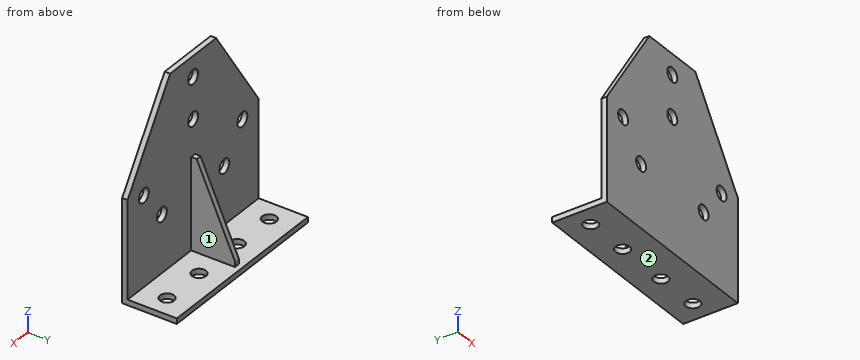
from build123d import *

# Parameters (mm, degrees)
SKETCH1_W      = 410
SKETCH1_H      = 120
SKETCH1_R      = 15.5
EXTRUDE1_DEPTH = 12
SKETCH2_W      = 410
SKETCH2_H      = 12
EXTRUDE2_DEPTH = 413
SKETCH3_R      = 15.5
EXTRUDE3_DEPTH = 413
SKETCH4_W      = 12
SKETCH4_H      = 96
EXTRUDE4_DEPTH = 200
EXTRUDE5_DEPTH = 200


with BuildPart() as part:
    # Sketch1 → Extrude1 (new body)
    with BuildSketch(Plane.XY):
        with Locations((205, 60)):
            Rectangle(SKETCH1_W, SKETCH1_H)
        with Locations((45, 67)):
            Circle(SKETCH1_R, mode=Mode.SUBTRACT)
        with Locations((145, 67)):
            Circle(SKETCH1_R, mode=Mode.SUBTRACT)
        with Locations((265, 67)):
            Circle(SKETCH1_R, mode=Mode.SUBTRACT)
        with Locations((365, 67)):
            Circle(SKETCH1_R, mode=Mode.SUBTRACT)
    extrude(amount=EXTRUDE1_DEPTH)

    # Sketch2 → Extrude2 (add)
    with BuildSketch(Plane.XY.offset(12)):
        with Locations((205, 6)):
            Rectangle(SKETCH2_W, SKETCH2_H)
    extrude(amount=EXTRUDE2_DEPTH)

    # Sketch3 → Extrude3 (cut)
    with BuildSketch(Plane(origin=(0, 12, 0), x_dir=(1, 0, 0), z_dir=(0, 1, 0))):
        with Locations(Location((302.738221798, -137.586347917, 0), (0, 0, 270))):
            Circle(SKETCH3_R)
        with Locations(Location((359.125657451, -207.732317869, 0), (0, 0, 270))):
            Circle(SKETCH3_R)
        with Locations(Location((107.261778202, -137.586347917, 0), (0, 0, 270))):
            Circle(SKETCH3_R)
        with Locations(Location((50.874342549, -207.732317869, 0), (0, 0, 270))):
            Circle(SKETCH3_R)
        with Locations(Location((205, -380, 0), (0, 0, 270))):
            Circle(SKETCH3_R)
        with Locations(Location((205, -290, 0), (0, 0, 270))):
            Circle(SKETCH3_R)
        Polygon((0, -425), (133, -425), (0, -225), align=None)
        Polygon((410, -425), (277, -425), (410, -225), align=None)
    extrude(amount=-EXTRUDE3_DEPTH, mode=Mode.SUBTRACT)

    # Sketch4 → Extrude4 (add)
    with BuildSketch(Plane.XY.offset(12)):
        with Locations((205, 60)):
            Rectangle(SKETCH4_W, SKETCH4_H)
    extrude(amount=EXTRUDE4_DEPTH)

    # Sketch5 → Extrude5 (cut)
    with BuildSketch(Plane.ZY.offset(-199)):
        Polygon((212, 108), (212, 24), (24, 108), align=None)
    extrude(amount=-EXTRUDE5_DEPTH, mode=Mode.SUBTRACT)


solid = part.part
Verification items for the finished model (mm, model axes). Face numbers are marked on the shaded views. A direction names the side the tool comes from. Give positions to 0.01 mm unless a question says otherwise; leave off trailing zeros. Loops run counter-clockwise (first coordinate to the right, second up) from the corner with the lowest first, then second, coordinate; pieces in that order, holes last.
1) Sectioned sample at D-D, the plane y = 42. Enter the section's corners in (x, z).
2) Thickness scan on line 1 along X through (y, z) = (11, 129); line 2 along Y through (x, z) = (270, 26); line 3 along X through (y, z) = (8, 144). Record the ranges inside material, lowest first.
3) Depth check by flat-ended pin: pin 1 Ø3.5 at (x, z) = (207.5, 17) entering from +Y; pin 2 Ø1 at (x, y) = (84, 20.5) entering from +Z; pin 3 Ø5 at (x, z) = (116, 217.5) entering from +Y. Enter the tip coordinate at first touch or a pass-through.
4) Set-up check for the marked faces 1 and 2: record each of +Z, -Z, +X, -X, +Y, -Y from which the full face is reachable in a straight line by a thin tool's end or side.
5) Sectioned sample at B-B, the plane z = 380. Enter the section's corners in (x, y) (3 decimals), then the cut area to 3 significant figures.
6) Sectioned sample at C-C, the plane x = 266.5. Enter the section's corners in (y, z), then the cut area to 3 significant figures.
7) Sectioned sample at A-A, the plane x = 205. Enter the section's corners in (y, z), then the cut area to 3 significant figures.
Answers:
1. outline: (0, 0) - (410, 0) - (410, 12) - (211, 12) - (211, 171.71) - (199, 171.71) - (199, 12) - (0, 12) - close
2. line 1: x = 0 to 94.36, 120.17 to 289.83, 315.64 to 410
2. line 2: y = 0 to 12
2. line 3: x = 0 to 93.15, 121.37 to 288.63, 316.85 to 410
3. pin 1: stops at y = 108
3. pin 2: stops at z = 12
3. pin 3: stops at y = 12
4. face 1: +Z, +X, +Y
4. face 2: -Z, +X, -X, +Y, -Y
5. outline: (103.075, 0) - (189.5, 0) - (189.5, 12) - (103.075, 12) - close; (220.5, 0) - (306.925, 0) - (306.925, 12) - (220.5, 12) - close
5. area: 2,070 mm2
6. outline: (0, 0) - (51.57, 0) - (51.57, 12) - (12, 12) - (12, 425) - (0, 425) - close; (82.43, 0) - (120, 0) - (120, 12) - (82.43, 12) - close
6. area: 6,030 mm2
7. outline: (0, 0) - (120, 0) - (120, 12) - (108, 12) - (108, 24) - (24, 212) - (12, 212) - (12, 274.5) - (0, 274.5) - close; (0, 305.5) - (12, 305.5) - (12, 364.5) - (0, 364.5) - close; (0, 395.5) - (12, 395.5) - (12, 425) - (0, 425) - close
7. area: 17,000 mm2
